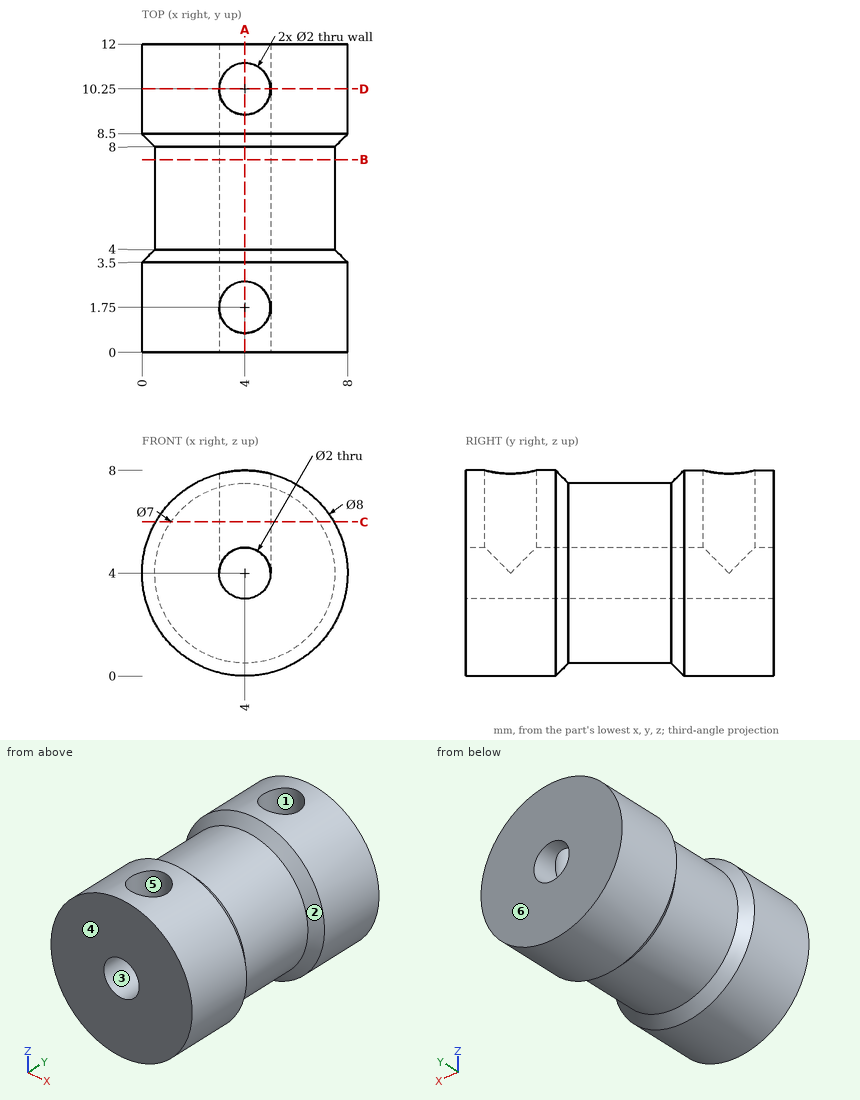
Part print with two shaded views. Sizes in mm from the minimum x, y, z corner. A direction names the side the tool comes from. Give positions to 0.01 mm unless a question says otherwise; leave off trailing zeros. Order: outer loops, then holes, each group sorted by start corner. A loop starts at its lowest first (then second) coordinate and runs counter-clockwise, first axis right, second up. Notation, with made-up numbers: (56, 67.5) - (93, 67.5) arc R11 cw to (93, 79.5) - close; hole circle Ø4 at (3, 64.25). An arc over 180 degrees is marked (long way). Write each question's results on one line, items separated by ' | '.
1. Pull direction Y, two halves, no side cores. Call the marked faces 4, 5 and 6: released by +Y, released by -Y, zero draft, split by the parting line, or undercut.
Calculated:
face 4: released by -Y | face 5: undercut | face 6: released by +Y
2. Pin check, flat tips, straight feed: pin 1 (4 mm diameter, centred on x = 6.5, y = 8, fed in from +Z); pin 2 (1 mm diameter, centred on y = 8.5, z = 5.5, fed in from +X); pin 3 (1.8 mm diameter, centred on x = 4, z = 4, fed in from -Y); pin 4 (3 mm diameter, centred on x = 6.5, y = 2.5, fed in from -Z). Stop position of each tip, or through.
Calculated:
pin 1: stops at z = 7.96 | pin 2: stops at x = 7.87 | pin 3: passes through | pin 4: stops at z = 0.13
3. Saw through at D-D on y = 10.25. List the corners of the cut face in (x, z), and give its area (3 significant figures).
Calculated:
outline: (3, 4) - (3, 7.87) arc R4 ccw (long way) to (5, 7.87) - (5, 4) arc R1 cw to start | area: 40.8 mm2
4. Saw through at B-B on y = 7.5. List the corners of the cut face in (x, z).
Calculated:
outline: circle Ø7 at (4, 4); hole circle Ø2 at (4, 4)
5. 3-axis set-ups, long thin cutter, end or side, ignore diameter. For the marked faces 1, 2 and 3: which of +Z, -Z, +X, -X, +Y, -Y reach the whole face in a straight line?
Calculated:
face 1: +Z | face 2: none | face 3: +Y, -Y
6. Saw through at A-A on x = 4. List the corners of the cut face in (y, z).
Calculated:
outline: (0, 0) - (3.5, 0) - (4, 0.5) - (8, 0.5) - (8.5, 0) - (12, 0) - (12, 3) - (0, 3) - close; (0, 5) - (0.75, 5) - (0.75, 8) - (0, 8) - close; (2.75, 5) - (9.25, 5) - (9.25, 8) - (8.5, 8) - (8, 7.5) - (4, 7.5) - (3.5, 8) - (2.75, 8) - close; (11.25, 5) - (12, 5) - (12, 8) - (11.25, 8) - close
7. Probe L1, parallel to Y at x = 4.25, z = 5.5; L2, parallel to X at y = 1.75, z = 7.15; L3, parallel to Z at x = 4.75, y = 11.25. List the from-to ranges inside material, lowest first. Write a range as from..to.
Calculated:
L1: y = 0..0.78, 2.72..9.28, 11.22..12 | L2: x = 1.53..3, 5..6.47 | L3: z = 0.07..3.34, 4.66..7.93
8. Saw through at C-C on z = 6. Count the separate pieces of the cut face and the enclosed holes in it, and give its area (3 significant figures).
Calculated:
separate pieces: 1 | enclosed holes: 2 | area: 71.5 mm2
